```python
from build123d import *

# Parameters (mm, degrees)
BOSS_EXTRUDE1_DEPTH                                 = 37.5
CHAMFER1_SIZE                                       = 18
CHAMFER2_SIZE                                       = 2
CSK_FOR_M4_COUNTERSUNK_FLAT_HEAD_SCREW1_D           = 4.5
CSK_FOR_M4_COUNTERSUNK_FLAT_HEAD_SCREW1_CSINK_D     = 9.4
CSK_FOR_M4_COUNTERSUNK_FLAT_HEAD_SCREW1_CSINK_ANGLE = 90


with BuildPart() as part:
    # Sketch1 → Boss-Extrude1 (new, symmetric)
    with BuildSketch(Plane(origin=(0, 0, 0), x_dir=(1, 0, 0), z_dir=(0, 1, 0))):
        Polygon((-9, 1), (9, 1), (9, 0), (11, 0), (11, 4), (4.1, 4), (4.1, 13), (9, 13), (9, 18), (-9, 18), (-9, 13), (-4.1, 13), (-4.1, 4), (-11, 4), (-11, 0), (-9, 0), align=None)
    extrude(amount=BOSS_EXTRUDE1_DEPTH, both=True)

    # Chamfer1
    # the kernel refuses this chamfer: 18 mm, written as the material it takes off along each edge
    with BuildSketch(Plane(origin=(55.290293783, -37.5, -18), x_dir=(0, 0.9996219169112966, -0.02749587661058639), z_dir=(-1, 0, 0))) as chamfer1_piece_1:
        Polygon((CHAMFER1_SIZE * 0.999621916911, -CHAMFER1_SIZE * 0.0274958766106), (-CHAMFER1_SIZE * 0.0274958766106, -CHAMFER1_SIZE * 0.999621916911), (0, 0), align=None)
    extrude(amount=110.580587567, mode=Mode.SUBTRACT)
    with BuildSketch(Plane(origin=(55.290293783, 37.5, -18), x_dir=(0, -0.9996219169112966, -0.02749587661058639), z_dir=(-1, 0, 0))) as chamfer1_piece_2:
        Polygon((CHAMFER1_SIZE * 0.999621916911, CHAMFER1_SIZE * 0.0274958766106), (-CHAMFER1_SIZE * 0.0274958766106, CHAMFER1_SIZE * 0.999621916911), (0, 0), align=None)
    extrude(amount=110.580587567, mode=Mode.SUBTRACT)

    # Chamfer2
    chamfer2_edges = [part.edges().sort_by_distance(p)[0] for p in [
        (-9, 0, -18),
        (9, 0, -18),
    ]]
    chamfer(chamfer2_edges, length=CHAMFER2_SIZE)

    # CSK for M4 Countersunk Flat Head Screw1 (through all)
    with Locations(Plane(origin=(0, 0, -18), x_dir=(-1, 0, 0), z_dir=(0, 0, -1))):
        with Locations((0, 14), (0, -14)):
            CounterSinkHole(CSK_FOR_M4_COUNTERSUNK_FLAT_HEAD_SCREW1_D / 2, CSK_FOR_M4_COUNTERSUNK_FLAT_HEAD_SCREW1_CSINK_D / 2, counter_sink_angle=CSK_FOR_M4_COUNTERSUNK_FLAT_HEAD_SCREW1_CSINK_ANGLE)


solid = part.part
```
Verification items for the finished model (mm, model axes). A direction names the side the tool comes from. Coordinates: 2 decimals unless noted, no trailing zeros. Loops run counter-clockwise (first coordinate to the right, second up) from the corner with the lowest first, then second, coordinate; pieces in that order, holes last. Notation, with made-up numbers: (87.25, 30.5) - (112.25, 30.5) arc R28 ccw to (112.25, 62.5) - close; hole circle Ø9 at (-19.5, 26.25). An arc over 180 degrees is marked (long way). Return JSON: item names as keys, results as strings.
1. Thickness scan on L1, parallel to Y at x = 0, z = -8.25; L2, parallel to Y at x = 0.5, z = -12.25; L3, parallel to X at y = 14, z = -9.75. Record the ranges inside material, lowest first.
Established:
{"L1": "y = -29.25 to -16.25, -11.75 to 11.75, 16.25 to 29.25", "L2": "y = -25.25 to -16.19, -11.81 to 11.81, 16.19 to 25.25", "L3": "x = -4.1 to -2.25, 2.25 to 4.1"}
2. Go/stop test with flat-tipped pins: pin 1 (4.5 mm diameter, centred on y = -15.5, z = -10, fed in from +X); pin 2 (3 mm diameter, centred on x = 4.5, y = 25, fed in from -Z); pin 3 (2 mm diameter, centred on x = 5, z = -13.5, fed in from +Y). Record where each tip stops, or that it passes through.
Established:
{"pin 1": "stops at x = 4.1", "pin 2": "stops at z = -14", "pin 3": "stops at y = 24.5"}
3. Mould release check, pull along Z, two halves, no side actions. Record for faces 1 (the flat face through (-10, 1, 0)), 2 (the conical face through (1.093, -16.102, -15.669)), 3 (the flat face through (-7, 0, -13)): +Z half, -Z half, draft (parallel to the pull), parting line (faces both ways), or undercut.
Established:
{"face 1": "+Z half", "face 2": "-Z half", "face 3": "undercut"}
4. Tool access check on faces 4 (the flat face through (-8, 0, -4)), 5 (the flat face through (0, 1, -1)), 6 (the flat face through (8, 0, -4)). Record the directions out of +Z, -Z, +X, -X, +Y, -Y that give a thin tool (end or side, any length) a straight path to the whole face; none if there is none.
Established:
{"face 4": "-X, +Y, -Y", "face 5": "+Z, +Y, -Y", "face 6": "+X, +Y, -Y"}
5. Section check D-D, the plane x = 0. Record the boundary of the cut face in (y, z), then the cut area to 3 significant figures.
Established:
{"outline": "(-36.5, -1) - (-19.5, -18) - (-18.7, -18) - (-16.25, -15.55) - (-16.25, -1) - close; (-11.75, -15.55) - (-9.3, -18) - (9.3, -18) - (11.75, -15.55) - (11.75, -1) - (-11.75, -1) - close; (16.25, -15.55) - (18.7, -18) - (19.5, -18) - (36.5, -1) - (16.25, -1) - close", "area": "787 mm2"}
6. Section check A-A, the plane y = 14. Record the boundary of the cut face in (x, z).
Established:
{"outline": "(-11, -4) - (-4.1, -4) - (-4.1, -13) - (-9, -13) - (-9, -16) - (-7, -18) - (-4.7, -18) - (-2.25, -15.55) - (-2.25, -1) - (-9, -1) - (-9, 0) - (-11, 0) - close; (2.25, -15.55) - (4.7, -18) - (7, -18) - (9, -16) - (9, -13) - (4.1, -13) - (4.1, -4) - (11, -4) - (11, 0) - (9, 0) - (9, -1) - (2.25, -1) - close"}
7. Section check B-B, the plane x = 8. Record the boundary of the cut face in (y, z), then the cut area to 3 significant figures.
Established:
{"outline": "(-36.5, -1) - (-33.5, -4) - (33.5, -4) - (36.5, -1) - close; (-24.5, -13) - (-20.5, -17) - (20.5, -17) - (24.5, -13) - close", "area": "390 mm2"}
8. Section check C-C, the plane y = 25.5. Record the boundary of the cut face in (x, z).
Established:
{"outline": "(-11, -4) - (-4.1, -4) - (-4.1, -12) - (4.1, -12) - (4.1, -4) - (11, -4) - (11, 0) - (9, 0) - (9, -1) - (-9, -1) - (-9, 0) - (-11, 0) - close"}
